Autodesk Inventor part; units mm, degrees
ref_plane "YZ Plane" through (0, 0, 0) normal (1, 0, 0) x (0, 1, 0)
ref_plane "XZ Plane" through (0, 0, 0) normal (0, 1, 0) x (-1, 0, 0)
ref_plane "XY Plane" through (0, 0, 0) normal (0, 0, 1) x (1, 0, 0)
sketch "Sketch1" plane through (0, 0, 0) normal (0, 1, 0) x (-1, 0, 0)
  circle A0 centre (0, 0) radius 1.5
  circle A1 centre (0, 0) radius 2.5
  line L0 (0, 0) -> (2.5, 0)
  line L1 (0, 0.75) -> (2.5, 0.75)
  line L2 (0, -0.75) -> (2.5, -0.75)
  line L3 (0, 2.5) -> (-2.5, 2.5)
  line L4 (-2.5, 2.5) -> (-2.5, -2.5)
  line L5 (-2.5, -2.5) -> (0, -2.5)
  line L6 (0, -2.5) -> (0, 2.5)
  point P0 (1.299, 0.75)
  point P1 (2.3848, 0.75)
  point P2 (2.3848, -0.75)
  point P3 (1.299, -0.75)
  dimension "d0" = 3
  dimension "d1" = 5
  dimension "d2" = 0.75
  dimension "d3" = 0.75
extrude "Extrusion1" add sketch "Sketch1" along normal blind 2 contours L0 A1 L2 A0 | A0 L1 A1 L0 | A0 L6 A1 L1 | L2 A1 L6 A0 | A0 L6 A1 | A1 L4 L3 | L5 L4 A1
sketch "Sketch2" plane through (2.5, 0, 2.5) normal (1, 0, 0) x (0, 0, -1)
  line L0 (1, 1.5) -> (4, 1.5)
  line L1 (4, 1.5) -> (4, 0.5)
  line L2 (4, 0.5) -> (1, 0.5)
  line L3 (1, 0.5) -> (1, 1.5)
  line L4 (0, 0) -> (5, 0)
  line L5 (5, 0) -> (5, 2)
  point P0 (2.5, 0)
  dimension "d6" = 3
  dimension "d7" = 1
  dimension "d8" = 0.5
  dimension "d9" = 1
extrude "Extrusion2" add sketch "Sketch2" along normal blind 1.5
properties part number "AlignmentGateClosed"
CAD build for the part. Positions are in the model's coordinates, mm. A direction names the side the tool comes from. Round coordinates to 2 decimals unless told otherwise and drop trailing zeros. Write each loop counter-clockwise with the first axis right and the second up, starting at its lowest first coordinate (ties: lowest second). Pieces come first, ordered by that corner, then holes. Notation, with made-up numbers: (47, 69) -> (105, 69) arc R17 ccw to (105, 89) -> close; hole circle Ø1 at (13.25, -0.5). An arc over 180 degrees is marked (long way). Answer as a JSON object with one key per item and string values.
(1) Which spindle directions (+Z, -Z, +X, -X, +Y, -Y) get a long thin tool onto all of the face, cutting with end or side? Do faces 5 (the face through (4, 1, 0)), 6 (the face through (3, 0.5, 0)), 7 (the face through (3, 1.5, 0)), 8 (the face through (1, 1, 2.5)), 9 (the face through (3, 1, -1.5)). Say none if no direction does.
Reported:
{"face 5": "+Z, -Z, +X, +Y, -Y", "face 6": "+Z, -Z, +X, -Y", "face 7": "+Z, -Z, +X, +Y", "face 8": "+Z, +X, -X, +Y, -Y", "face 9": "-Z, +X, +Y, -Y"}
(2) Band-saw the part on A-A, the plane z = 0. List the corners of the cut face in (x, y), then the cut area to 3 significant figures.
Reported:
{"outline": "(-2.5, 0) -> (-1.5, 0) -> (-1.5, 2) -> (-2.5, 2) -> close; (1.5, 0) -> (2.5, 0) -> (2.5, 0.5) -> (4, 0.5) -> (4, 1.5) -> (2.5, 1.5) -> (2.5, 2) -> (1.5, 2) -> close", "area": "5.50 mm^2"}
(3) Probe probe 1 along X at (y, z) = (1, 0); probe 2 along X at (y, z) = (0.3, 0). List the from-to ranges inside material, lowest first. Write a range as [from, to].
Reported:
{"probe 1": "x = [-2.5, -1.5], [1.5, 4]", "probe 2": "x = [-2.5, -1.5], [1.5, 2.5]"}
(4) Two-plate mould, pull along Z, no slides. Class faces 1 (the face through (-2.5, 1, 0.1)), 2 (the face through (2, 2, 0)), 3 (the face through (1.5, 0.99, -0.07)), 4 (the face through (3, 1, 1.5)): +Z half, -Z half, draft (parallel to the pull), parting line (faces both ways), or undercut.
Reported:
{"face 1": "parting line", "face 2": "draft", "face 3": "undercut", "face 4": "+Z half"}
(5) Band-saw the part on B-B, the plane y = 1.4. List the corners of the cut face in (x, z), then the cut area to 3 significant figures.
Reported:
{"outline": "(0, -2.5) -> (2.5, -2.5) -> (2.5, -1.5) -> (4, -1.5) -> (4, 1.5) -> (2.5, 1.5) -> (2.5, 2.5) -> (0, 2.5) arc R2.5 ccw to start; hole circle Ø3 at (0, 0)", "area": "19.7 mm^2"}
(6) Band-saw the part on D-D, the plane z = -0.55. List the corners of the cut face in (x, y), then the cut area to 3 significant figures.
Reported:
{"outline": "(-2.44, 0) -> (-1.4, 0) -> (-1.4, 2) -> (-2.44, 2) -> close; (1.4, 0) -> (2.5, 0) -> (2.5, 0.5) -> (4, 0.5) -> (4, 1.5) -> (2.5, 1.5) -> (2.5, 2) -> (1.4, 2) -> close", "area": "5.80 mm^2"}
(7) Pin check, flat tips, straight feed: P1, Ø1.6, axis at x = 3.5, z = 0, coming from the -Y side; P2, Ø0.8, axis at x = 3, y = 1, coming from the -Z side; P3, Ø3, axis at x = -1, z = -1, coming from the -Y side; P4, Ø1.2, axis at x = 3.5, z = -0.5, coming from the +Y side. Stop position of each tip, or through.
Reported:
{"P1": "stops at y = 0.5", "P2": "stops at z = -1.5", "P3": "stops at y = 0", "P4": "stops at y = 1.5"}
(8) Band-saw the part on C-C, the plane x = 0.25. List the corners of the cut face in (y, z).
Reported:
{"outline": "(0, -2.5) -> (2, -2.5) -> (2, -1.48) -> (0, -1.48) -> close; (0, 1.48) -> (2, 1.48) -> (2, 2.5) -> (0, 2.5) -> close"}
